Check sheet for the modelled part. Datum: model origin and axes. Units: mm. Give positions to 0.01 mm unless a question says otherwise; leave off trailing zeros. Order: outer loops, then holes, each group sorted by start corner. A loop starts at its lowest first (then second) coordinate and runs counter-clockwise, first axis right, second up. Notation, with made-up numbers: (51.25, 57) -> (78.25, 57) arc R14 ccw to (78.25, 72) -> close; hole circle Ø10 at (19, 37.5). An arc over 180 degrees is marked (long way). Answer in a Markdown table with one row per item. Add a question column.
(1) Go/stop test with flat-tipped pins: pin 1 (0.9 mm diameter, centred on x = 90.5, y = 1.5, fed in from +Z); pin 2 (1.5 mm diameter, centred on y = 1, z = -94, fed in from +X); pin 3 (1.5 mm diameter, centred on x = -88, y = 2, fed in from -Z). Record where each tip stops, or that it passes through.
(2) Cross-section at C-C (z = -36). Record the cut outline in (x, y), then the cut area to 3 significant figures.
(3) Cross-section at A-A (z = 0). Record the cut outline in (x, y), then the cut area to 3 significant figures.
(4) Cross-section at D-D (x = 54). Record the cut outline in (y, z), then the cut area to 3 significant figures.
(5) Cross-section at B-B (y = 0.65). State how many separate pieces and enclosed holes the cut face has, then the cut area to 3 significant figures.
(6) Thickness scan on L1, parallel to X at y = 2.15, z = 0.5; L2, parallel to Z at x = 70, y = 0.8; L3, parallel to X at y = 0.5, z = 8.5. Record the ranges inside material, lowest first. Write a range as [from, to].
Autodesk Inventor part; units mm, degrees
ref_plane "YZ Plane" through (0, 0, 0) normal (1, 0, 0) x (0, 1, 0)
ref_plane "XZ Plane" through (0, 0, 0) normal (0, 1, 0) x (-1, 0, 0)
ref_plane "XY Plane" through (0, 0, 0) normal (0, 0, 1) x (1, 0, 0)
sketch "Sketch1" plane through (0, 0, 0) normal (0, 1, 0) x (-1, 0, 0)
  circle A0 centre (0, 0) radius 125
  circle A1 centre (70, -90) radius 1.5
  circle A2 centre (-70, -90) radius 1.5
  circle A3 centre (-70, 90) radius 1.5
  circle A4 centre (70, 90) radius 1.5
  circle A5 centre (70, -70) radius 2
  circle A6 centre (-70, -70) radius 2
  circle A7 centre (-70, 70) radius 2
  circle A8 centre (70, 70) radius 2
  line L0 (5, -104.4418) -> (-5.5, -104.4418)
  line L1 (-5.5, -82.9418) -> (-5.5, -104.4418)
  line L2 (-5, -82.4418) -> (5.5, -82.4418)
  line L3 (5.5, -103.9418) -> (5.5, -82.4418)
  line L4 (-5, -82.4418) -> (-5.5, -82.4418)
  line L5 (-5.5, -82.4418) -> (-5.5, -82.9418)
  line L6 (5.5, -103.9418) -> (5.5, -104.4418)
  line L7 (5.5, -104.4418) -> (5, -104.4418)
  arc A9 (0.75, -108.2408) -> (-0.75, -108.2408) centre (0, -106.9418) ccw
  arc A10 (-0.75, -78.6427) -> (0.75, -78.6427) centre (0, -79.9418) ccw
  circle A11 centre (0, -106.9418) radius 1.5
  circle A12 centre (0, -79.9418) radius 1.5
  line L8 (98, 50) -> (82, 50)
  line L9 (80, 48) -> (80, -48)
  line L10 (82, -50) -> (98, -50)
  line L11 (100, -48) -> (100, 48)
  line L12 (-98, 50) -> (-82, 50)
  line L13 (-80, 48) -> (-80, -48)
  line L14 (-82, -50) -> (-98, -50)
  line L15 (-100, -48) -> (-100, 48)
  arc A13 (98, -50) -> (100, -48) centre (98, -48) ccw
  arc A14 (100, 48) -> (98, 50) centre (98, 48) ccw
  arc A15 (82, 50) -> (80, 48) centre (82, 48) ccw
  arc A16 (80, -48) -> (82, -50) centre (82, -48) ccw
  arc A17 (-82, -50) -> (-80, -48) centre (-82, -48) ccw
  arc A18 (-80, 48) -> (-82, 50) centre (-82, 48) ccw
  arc A19 (-98, 50) -> (-100, 48) centre (-98, 48) ccw
  arc A20 (-100, -48) -> (-98, -50) centre (-98, -48) ccw
  point P0 (0.75, -108.2408)
  point P1 (-0.75, -78.6427)
  point P2 (0.75, -78.6427)
  point P3 (-90, 0)
extrude "Extrusion6" add sketch "Sketch1" along normal blind 3
Answer below:
| question | item | result |
|---|---|---|
| 1 | pin 1 | stops at z = 86.69 |
| 1 | pin 2 | stops at x = 83.24 |
| 1 | pin 3 | stops at z = -89.51 |
| 2 | outline | (-119.7, 0) -> (-100, 0) -> (-100, 3) -> (-119.7, 3) -> close; (-80, 0) -> (80, 0) -> (80, 3) -> (-80, 3) -> close; (100, 0) -> (119.7, 0) -> (119.7, 3) -> (100, 3) -> close |
| 2 | area | 598 mm² |
| 3 | outline | (-125, 0) -> (-100, 0) -> (-100, 3) -> (-125, 3) -> close; (-80, 0) -> (80, 0) -> (80, 3) -> (-80, 3) -> close; (100, 0) -> (125, 0) -> (125, 3) -> (100, 3) -> close |
| 3 | area | 630 mm² |
| 4 | outline | (0, -112.73) -> (3, -112.73) -> (3, 112.73) -> (0, 112.73) -> close |
| 4 | area | 676 mm² |
| 5 | separate pieces | 1 |
| 5 | enclosed holes | 13 |
| 5 | area | 44,800 mm² |
| 6 | L1 | x = [-125, -100], [-80, 80], [100, 125] |
| 6 | L2 | z = [-103.56, -91.5], [-88.5, -72], [-68, 68], [72, 88.5], [91.5, 103.56] |
| 6 | L3 | x = [-124.71, -100], [-80, 80], [100, 124.71] |
